Input: part model. Units: mm. Frame: model coordinates. Face numbers are marked on the shaded views. A direction names the side the tool comes from. Round coordinates to 2 decimals unless told otherwise and drop trailing zeros. Loops run counter-clockwise (first coordinate to the right, second up) from the corner with the lowest first, then second, coordinate; pieces in that order, holes last. Notation, with made-up numbers: (71.25, 0) - (91.25, 0) arc R35 cw to (91.25, 36) - close; hole circle Ø10 at (49.25, -5.5). An arc over 180 degrees is marked (long way). Write each question's results on one line, items separated by ' | '.
from build123d import *

# Parameters (mm, degrees)
SKETCH033_W     = 131
SKETCH033_H     = 30
PAD012_DEPTH    = 10
SKETCH032_W     = 15
SKETCH032_H     = 30
PAD011_DEPTH    = 18.5
SKETCH030_W     = 30
SKETCH030_H     = 13.5
POCKET020_DEPTH = 10
SKETCH031_R     = 3
POCKET021_DEPTH = 10.001
SKETCH034_W     = 32.5
SKETCH034_H     = 30
POCKET022_DEPTH = 5
SKETCH040_R     = 5
POCKET028_DEPTH = 3
CHAMFER_SIZE2   = 25
CHAMFER_SIZE    = 10
CHAMFER010_SIZE = 1


with BuildPart() as part:
    # Sketch033 → Pad012 (new body)
    with BuildSketch(Plane.XY):
        Rectangle(SKETCH033_W, SKETCH033_H)
    extrude(amount=PAD012_DEPTH)

    # Sketch032 (on Face5 of Pad012) → Pad011 (join)
    with BuildSketch(Plane(origin=(0, 0, 0), x_dir=(1, 0, 0), z_dir=(0, 0, -1))):
        with Locations((-58, 0)):
            Rectangle(SKETCH032_W, SKETCH032_H)
    extrude(amount=PAD011_DEPTH)

    # Sketch030 (on Face9 of Pad011) → Pocket020 (cut)
    with BuildSketch(Plane.YZ.offset(-50.5)):
        with Locations((0, -6.75)):
            Rectangle(SKETCH030_W, SKETCH030_H)
    extrude(amount=-POCKET020_DEPTH, mode=Mode.SUBTRACT)

    # Sketch031 (on Face5 of Pocket020) → Pocket021 (cut, through all)
    with BuildSketch(Plane(origin=(0, 0, 0), x_dir=(1, 0, 0), z_dir=(0, 0, -1))):
        with Locations((50.5, 0)):
            Circle(SKETCH031_R)
    extrude(amount=-POCKET021_DEPTH, mode=Mode.SUBTRACT)

    # Sketch034 → Pocket022 (cut)
    with BuildSketch(Plane.XY.offset(10)):
        with Locations((49.25, 0)):
            Rectangle(SKETCH034_W, SKETCH034_H)
    extrude(amount=-POCKET022_DEPTH, mode=Mode.SUBTRACT)

    # Sketch040 (on Face4 of Pocket022) → Pocket028 (cut)
    with BuildSketch(Plane(origin=(0, 0, 0), x_dir=(1, 0, 0), z_dir=(0, 0, -1))):
        with Locations((50.5, 0)):
            Circle(SKETCH040_R)
    extrude(amount=-POCKET028_DEPTH, mode=Mode.SUBTRACT)

    # Chamfer
    chamfer_edges = [part.edges().sort_by_distance(p)[0] for p in [
        (-50.5, 15, -16),
    ]]
    chamfer_side = part.faces().sort_by_distance((-55.5, 15, -13.73817))[0]
    chamfer(chamfer_edges, length=CHAMFER_SIZE, length2=CHAMFER_SIZE2, reference=chamfer_side)

    # Chamfer010
    chamfer010_edges = [part.edges().sort_by_distance(p)[0] for p in [
        (-55.5, 2.5, -18.5),
        (-55.5, 2.5, -13.5),
        (-50.5, -12.5, -18.5),
        (-50.5, -12.5, -13.5),
        (-58, -15, -18.5),
        (-65.5, 0, -18.5),
        (-63, 15, -18.5),
        (-65.5, -15, -9.25),
        (-65.5, -15, 5),
        (-65.5, 0, 10),
        (-65.5, 15, 5),
        (-65.5, 15, -9.25),
    ]]
    chamfer(chamfer010_edges, length=CHAMFER010_SIZE)


solid = part.part
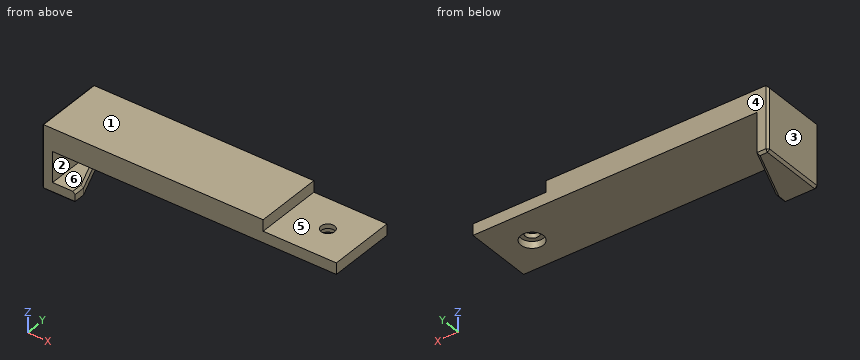
1. Contact query for flat-ended pins moving along their axis: pin 1 (2.5 mm diameter, centred on y = 5.5, z = 7, fed in from +X); pin 2 (8 mm diameter, centred on x = -36, y = 9, fed in from -Z); pin 3 (7 mm diameter, centred on x = 50.5, y = 0, fed in from -Z). Output: stop coordinate, or through.
Answer:
pin 1: x = 33 | pin 2: z = 0 | pin 3: z = 3
2. Set-up query: the marked faces 4, 5 and 6. Return all of +Z, -Z, +X, -X, +Y, -Y with unobstructed straight access to the full face (end or side cutting, diameter ignored); none if empty.
Answer:
face 4: +Z, -Z, +X, -X, +Y | face 5: +Z, +X, +Y, -Y | face 6: +X, +Y, -Y
3. Section query A-A, the plane x = 50.5. Output: boundary loops of the cut face in (y, z), plus the area to 3 significant figures.
Answer:
outline: (-15, 0) - (-5, 0) - (-5, 3) - (-3, 3) - (-3, 5) - (-15, 5) - close; (3, 3) - (5, 3) - (5, 0) - (15, 0) - (15, 5) - (3, 5) - close | area: 108 mm^2
4. Mould query, pull axis Z, two halves, no side actions, for the marked faces 1, 2 and 3. Classes: pulls with the +Z half, pulls with the -Z half, needs draft (parallel to the pull), parting line crosses it, or undercut.
Answer:
face 1: pulls with the +Z half | face 2: undercut | face 3: needs draft
5. Section query C-C, the plane z = -11.25. Output: boundary loops of the cut face in (x, y), plus the area to 3 significant figures.
Answer:
outline: (-65.5, -14) - (-64.5, -15) - (-60.5, -15) - (-60.5, 15) - (-64.5, 15) - (-65.5, 14) - close | area: 149 mm^2
6. Line query: line 1 (X direction, y = 0, z = 3.55); line 2 (Y direction, x = 50.5, z = 0.7); line 3 (X direction, y = 0, z = 1). Output: solid intervals per line, ascending. Write a range as [from, to].
Answer:
line 1: [-65.5, 47.5], [53.5, 65.5] | line 2: [-15, -5], [5, 15] | line 3: [-65.5, 45.5], [55.5, 65.5]
7. Section query D-D, the plane x = -37.5. Output: boundary loops of the cut face in (y, z), plus the area to 3 significant figures.
Answer:
outline: (-15, 0) - (15, 0) - (15, 10) - (-15, 10) - close | area: 300 mm^2
8. Section query B-B, the plane y = 0. Output: boundary loops of the cut face in (x, z), plus the area to 3 significant figures.
Answer:
outline: (-65.5, -17.5) - (-64.5, -18.5) - (-55.58, -18.5) - (-54.5, -17.5) - (-54.5, -14.5) - (-55.58, -13.5) - (-60.5, -13.5) - (-60.5, 0) - (45.5, 0) - (45.5, 3) - (47.5, 3) - (47.5, 5) - (33, 5) - (33, 10) - (-64.5, 10) - (-65.5, 9) - close; (53.5, 3) - (55.5, 3) - (55.5, 0) - (65.5, 0) - (65.5, 5) - (53.5, 5) - close | area: 1,230 mm^2
